from build123d import *

# Parameters (mm, degrees)
SKETCH1_W           = 55
SKETCH1_H           = 15
BOSS_EXTRUDE1_DEPTH = 3
SKETCH2_W           = 55
SKETCH2_H           = 3
BOSS_EXTRUDE2_DEPTH = 30
CUT_EXTRUDE1_DEPTH  = 30
SKETCH4_R           = 2.5
CUT_EXTRUDE2_DEPTH  = 30
BOSS_EXTRUDE3_DEPTH = 2
FILLET1_R           = 10
SKETCH6_W           = 15
SKETCH6_H           = 5
CUT_EXTRUDE3_DEPTH  = 10
FILLET2_R           = 2
FILLET3_R           = 2
FILLET4_R           = 2
FILLET5_R           = 5


with BuildPart() as part:
    # Sketch1 → Boss-Extrude1 (new body)
    with BuildSketch(Plane(origin=(0, 0, 0), x_dir=(1, 0, 0), z_dir=(0, 1, 0))):
        Rectangle(SKETCH1_W, SKETCH1_H)
    extrude(amount=BOSS_EXTRUDE1_DEPTH)

    # Sketch2 → Boss-Extrude2 (add)
    with BuildSketch(Plane(origin=(0, 3, 0), x_dir=(1, 0, 0), z_dir=(0, 1, 0))):
        with Locations((0, 6)):
            Rectangle(SKETCH2_W, SKETCH2_H)
    extrude(amount=BOSS_EXTRUDE2_DEPTH)

    # Sketch3 → Cut-Extrude1 (cut)
    with BuildSketch(Plane.XY.offset(-4.5)):
        with BuildLine():
            Line((-15.25, 26.2), (-10.25, 26.2))
            ThreePointArc((-10.25, 26.2), (-2.05, 18), (-10.25, 9.8))
            Line((-10.25, 9.8), (-15.25, 9.8))
            ThreePointArc((-15.25, 9.8), (-23.45, 18), (-15.25, 26.2))
        make_face()
        with BuildLine():
            Line((15.25, 26.2), (10.25, 26.2))
            ThreePointArc((10.25, 26.2), (2.05, 18), (10.25, 9.8))
            Line((10.25, 9.8), (15.25, 9.8))
            ThreePointArc((15.25, 9.8), (23.45, 18), (15.25, 26.2))
        make_face()
    extrude(amount=-CUT_EXTRUDE1_DEPTH, mode=Mode.SUBTRACT)

    # Sketch4 → Cut-Extrude2 (cut)
    with BuildSketch(Plane(origin=(0, 3, 0), x_dir=(1, 0, 0), z_dir=(0, 1, 0))):
        with Locations(Location((-15, -2.5, 0), (0, 0, 270))):
            Circle(SKETCH4_R)
        with Locations(Location((15, -2.5, 0), (0, 0, 270))):
            Circle(SKETCH4_R)
    extrude(amount=-CUT_EXTRUDE2_DEPTH, mode=Mode.SUBTRACT)

    # Sketch5 → Boss-Extrude3 (add)
    with BuildSketch(Plane.ZY.offset(27.5)):
        Polygon((7.5, 3), (-4.5, 3), (-4.5, 13), align=None)
    boss_extrude3 = extrude(amount=-BOSS_EXTRUDE3_DEPTH)

    # Mirror1: Boss-Extrude3 across plane
    add(boss_extrude3.mirror(Plane(origin=(0, 0, 0), x_dir=(0, 0, 1), z_dir=(1, 0, 0))))

    # Fillet1
    fillet1_edges = [part.edges().sort_by_distance(p)[0] for p in [
        (-27.5, 33, -6),
        (27.5, 33, -6),
    ]]
    fillet(fillet1_edges, radius=FILLET1_R)

    # Sketch6 → Cut-Extrude3 (cut)
    with BuildSketch(Plane(origin=(0, 0, -7.5), x_dir=(-1, 0, 0), z_dir=(0, 0, -1))):
        with Locations((0, 10.75)):
            Rectangle(SKETCH6_W, SKETCH6_H)
    extrude(amount=-CUT_EXTRUDE3_DEPTH, mode=Mode.SUBTRACT)

    # Fillet2
    # the kernel refuses this fillet: 2 mm, written as the material it takes off along each edge
    with BuildSketch(Plane(origin=(-7.5, 10.274878642, -12.896978856), x_dir=(0, -1, 0), z_dir=(0, 0, 1))) as fillet2_piece_1:
        with BuildLine():
            CenterArc((2.443897749, -1.9556132), FILLET2_R, 102.093612403, 82.373166868)
            Line((0.449972434, -2.111375318), (0.410093928, -2.11449056))
            ThreePointArc((0.410093928, -2.11449056), (0.255650409, -1.049152563), (-0.037683519, -0.013414634))
            Line((-0.037683519, -0.013414634), (0, 0.04))
            ThreePointArc((0, 0.04), (1.012439321, 0.04), (2.01649826, 0.039112264))
            Line((2.01649826, 0.039112264), (2.024878642, 0))
        make_face()
    extrude(amount=13.793957711, mode=Mode.SUBTRACT)
    with BuildSketch(Plane(origin=(7.5, 10.274878642, -12.896978856), x_dir=(0.9780357557406035, -0.2084371859647568, 0), z_dir=(0, 0, 1))) as fillet2_piece_2:
        with BuildLine():
            CenterArc((2.422058804, -1.98259687), FILLET2_R, 97.564003787, 82.373166868)
            Line((0.422060006, -1.980403713), (0.38206003, -1.980359849))
            ThreePointArc((0.38206003, -1.980359849), (0.171908573, -0.998539344), (-0.03912143, -0.008337487))
            Line((-0.03912143, -0.008337487), (0.005265345, 0.039651937))
            ThreePointArc((0.005265345, 0.039651937), (1.079395771, -0.031352833), (2.153526197, 0.039651937))
            Line((2.153526197, 0.039651937), (2.158791542, 0))
        make_face()
    extrude(amount=13.793957711, mode=Mode.SUBTRACT)

    # Fillet3
    fillet3_edges = [part.edges().sort_by_distance(p)[0] for p in [
        (-3.565877021, 13.25, -6),
        (3.565877021, 13.25, -6),
    ]]
    fillet(fillet3_edges, radius=FILLET3_R)

    # Fillet4
    fillet4_edges = [part.edges().sort_by_distance(p)[0] for p in [
        (-7.5, 8.25, -6),
        (7.5, 8.25, -6),
    ]]
    fillet(fillet4_edges, radius=FILLET4_R)

    # Fillet5
    # the kernel refuses this fillet: 5 mm, written as the material it takes off along each edge
    with BuildSketch(Plane(origin=(27.5, -12.5, 7.5), x_dir=(0, 0, -1), z_dir=(0, 1, 0))) as fillet5_piece_1:
        with BuildLine():
            CenterArc((FILLET5_R, FILLET5_R), FILLET5_R, 180, 90)
            Line((0, FILLET5_R), (0, 0))
            Line((0, 0), (FILLET5_R, 0))
        make_face()
    extrude(amount=28, mode=Mode.SUBTRACT)
    with BuildSketch(Plane(origin=(-27.5, -12.5, 7.5), x_dir=(0, 0, -1), z_dir=(0, 1, 0))) as fillet5_piece_2:
        with BuildLine():
            CenterArc((FILLET5_R, -FILLET5_R), FILLET5_R, 90, 90)
            Line((0, -FILLET5_R), (0, 0))
            Line((0, 0), (FILLET5_R, 0))
        make_face()
    extrude(amount=28, mode=Mode.SUBTRACT)


solid = part.part
Input: part model. Units: mm. Frame: model coordinates. A direction names the side the tool comes from. Give positions to 0.01 mm unless a question says otherwise; leave off trailing zeros. Order: outer loops, then holes, each group sorted by start corner. A loop starts at its lowest first (then second) coordinate and runs counter-clockwise, first axis right, second up. Notation, with made-up numbers: (5.25, 35.5) - (43.25, 35.5) arc R18 cw to (43.25, 50.5) - close; hole circle Ø10 at (47, 78). An arc over 180 degrees is marked (long way). Answer as a JSON object with one key per item and string values. Group by question number.
Q1. Cut plane C-C, the plane z = 3.5. Output: boundary loops of the cut face in (x, y).
Q2. Cut plane A-A, the plane y = 18. Output: boundary loops of the cut face in (x, z), then the cut area to 3 significant figures.
Q3. First-contact query: pin 1 Ø6 at (x, z) = (15, 2.5) entering from +Y; pin 2 Ø5 at (x, y) = (15.5, 14) entering from +Z. Flat tips, straight axial feed; report the tip coordinate or a pass-through.
Q4. Cut plane D-D, the plane y = 28. Output: boundary loops of the cut face in (x, z), then the cut area to 3 significant figures.
Q5. Cut plane B-B, the plane z = -1.5. Output: boundary loops of the cut face in (x, y).
Q6. Line query: probe 1 along X at (y, z) = (0.9, 2.5); probe 2 along Y at (x, z) = (-11.5, -5); probe 3 along Y at (x, z) = (-15.5, -1). Output: solid intervals per line, ascending.
Q7. Set-up query: faces 4 (the face through (-26.63, 2.74, 5.32)), 5 (the face through (-25.5, 7, 0)), 6 (the face through (-13, 26.2, -6)). Return all of +Z, -Z, +X, -X, +Y, -Y with unobstructed straight access to the full face (end or side cutting, diameter ignored); none if empty.
Q8. Mould query, pull axis Y, two halves, no side actions, for faces 1 (the face through (-26.5, 8.5, 0.9)), 2 (the face through (-27.5, 9, -4)), 3 (the face through (2.005, 14.021, -5.979)). Classes: pulls with the +Y half, pulls with the -Y half, needs draft (parallel to the pull), parting line crosses it, or undercut.
Results:
{
 "1": {"outline": "(-27.4, 0) - (-17.29, 0) - (-17.29, 3) - (-25.5, 3) - (-25.5, 6.33) - (-27.4, 6.33) - close; (-12.71, 0) - (12.71, 0) - (12.71, 3) - (-12.71, 3) - close; (17.29, 0) - (27.4, 0) - (27.4, 6.33) - (25.5, 6.33) - (25.5, 3) - (17.29, 3) - close"},
 "2": {"outline": "(-27.5, -7.5) - (-23.45, -7.5) - (-23.45, -4.5) - (-27.5, -4.5) - close; (-2.05, -7.5) - (2.05, -7.5) - (2.05, -4.5) - (-2.05, -4.5) - close; (23.45, -7.5) - (27.5, -7.5) - (27.5, -4.5) - (23.45, -4.5) - close", "area": "36.6 mm^2"},
 "3": {"pin 1": "y = 3", "pin 2": "through"},
 "4": {"outline": "(-26.16, -7.5) - (26.16, -7.5) - (26.16, -4.5) - (-26.16, -4.5) - close", "area": "157 mm^2"},
 "5": {"outline": "(-27.5, 0) - (27.5, 0) - (27.5, 10.5) - (25.5, 10.5) - (25.5, 3) - (-25.5, 3) - (-25.5, 10.5) - (-27.5, 10.5) - close"},
 "6": {"probe 1": "-27.5 to -17.5, -12.5 to 12.5, 17.5 to 27.5", "probe 2": "0 to 9.8, 26.2 to 33", "probe 3": "0 to 3"},
 "7": {"face 4": "+Z, -X, +Y, -Y", "face 5": "+Z, +Y", "face 6": "+Z, -Z"},
 "8": {"face 1": "pulls with the +Y half", "face 2": "needs draft", "face 3": "undercut"}
}
